Input: part model. Units: mm. Frame: model coordinates. A direction names the side the tool comes from. Give positions to 0.01 mm unless a question says otherwise; leave off trailing zeros. Loops run counter-clockwise (first coordinate to the right, second up) from the corner with the lowest first, then second, coordinate; pieces in that order, holes last. Notation, with made-up numbers: (-26.75, 72) - (21.25, 72) arc R21 ccw to (21.25, 105) - close; hole circle Ø7 at (9.5, 88). An arc over 180 degrees is marked (long way). Answer as a JSON object with one key per item and string values. Group by question number.
(1) Access query for faces 4 (the flat face through (1, 1, 0)), 5 (the flat face through (-4.6, -15.1, 9.6)). Directions: +Z, -Z, +X, -X, +Y, -Y. A direction counts if a zero-diameter tool reaches every point of the face in a straight line with its end or side. Return the directions, or none.
(2) Pin query (flat end, axial travel): P1, Ø5, axis at x = -3.5, y = -3, coming from the +Z side; P2, Ø3, axis at y = -4, z = 8, coming from the +X side; P3, Ø6, axis at y = -12, z = 15, coming from the -X side. Return the tip coordinate at first contact, or that it passes through.
(3) Section query B-B (z = 9.25). Return loops of the section in (x, y), plus the area to 3 significant figures.
(4) Section query A-A (x = 0). Return loops of the section in (y, z).
(5) Section query C-C (y = 2). Return loops of the section in (x, z), plus the area to 3 significant figures.
(6) Material intervals for L1, parallel to Z at x = 2, y = -5.25; L2, parallel to Z at x = 0.5, y = 1.75; L3, parallel to X at y = 0, z = -0.9, sorted ascending.
(7) Section query D-D (x = -7.5). Return loops of the section in (y, z), plus the area to 3 significant figures.
(8) Mould query, pull axis Y, two halves, no side actions, for faces 1 (the flat face through (0.468, -11.968, 6.703)), 2 (the flat face through (-1.494, 0.465, -1.578)), 3 (the flat face through (-2.26, -7.45, 12.51)). Classes: +Y half, -Y half, draft (parallel to the pull), parting line (faces both ways), or undercut.
```python
from build123d import *

# Parameters (mm, degrees)
SKETCH1_R           = 4
SKETCH1_R_2         = 2.3
BOSS_EXTRUDE1_DEPTH = 3.2
SKETCH2_R           = 4
SKETCH2_R_2         = 0.85
BOSS_EXTRUDE2_DEPTH = 2
BOSS_EXTRUDE3_DEPTH = 8
SKETCH6_R           = 0.85
CUT_EXTRUDE1_DEPTH  = 6.2


with BuildPart() as part:
    # Sketch1 → Boss-Extrude1 (new body)
    with BuildSketch(Plane.XY):
        Circle(SKETCH1_R)
        Circle(SKETCH1_R_2, mode=Mode.SUBTRACT)
    extrude(amount=-BOSS_EXTRUDE1_DEPTH)

    # Sketch2 → Boss-Extrude2 (add)
    with BuildSketch(Plane.XY):
        Circle(SKETCH2_R)
        Circle(SKETCH2_R_2, mode=Mode.SUBTRACT)
    extrude(amount=BOSS_EXTRUDE2_DEPTH)

    # Sketch5 → Boss-Extrude3 (add)
    with BuildSketch(Plane(origin=(3.819651946, -1.187543266, 0), x_dir=(0, 0, -1), z_dir=(0.954912987, -0.296885816, 0))):
        Polygon((-2, 0), (3.2, 0), (3.2, -15.784917441), (-22.731913212, -15.784917441), (-22.731913212, -7.784917441), (-2, -7.784917441), align=None)
    extrude(amount=-BOSS_EXTRUDE3_DEPTH)

    # Sketch6 → Cut-Extrude1 (cut, through all)
    with BuildSketch(Plane.XY.offset(2)):
        Circle(SKETCH6_R)
    extrude(amount=-CUT_EXTRUDE1_DEPTH, mode=Mode.SUBTRACT)


solid = part.part
```
Recorded:
{
 "1": {"face 4": "-Z", "face 5": "+Z, -Z, -X, -Y"},
 "2": {"P1": "stops at z = 2", "P2": "passes through", "P3": "stops at x = -8.51"},
 "3": {"outline": "(-8.51, -13.89) - (-0.87, -16.26) - (1.51, -8.62) - (-6.13, -6.25) - close", "area": "64.0 mm^2"},
 "4": {"outline": "(-13.47, -3.2) - (-0.85, -3.2) - (-0.85, 2) - (-8.15, 2) - (-8.15, 22.73) - (-13.47, 22.73) - close; (0.85, 0) - (2.3, 0) - (2.3, -3.2) - (4, -3.2) - (4, 2) - (0.85, 2) - close"},
 "5": {"outline": "(-3.46, -3.2) - (-1.14, -3.2) - (-1.14, 0) - (1.14, 0) - (1.14, -3.2) - (3.46, -3.2) - (3.46, 2) - (-3.46, 2) - close", "area": "28.8 mm^2"},
 "6": {"L1": "z = -3.2 to 2", "L2": "z = 0 to 2", "L3": "x = -4.19 to -0.85, 2.3 to 4"},
 "7": {"outline": "(-14.2, -3.2) - (-10.65, -3.2) - (-10.65, 22.73) - (-14.2, 22.73) - close", "area": "92.0 mm^2"},
 "8": {"face 1": "-Y half", "face 2": "undercut", "face 3": "+Y half"}
}
